```python
from build123d import *

# Parameters (mm, degrees)
SKETCH1_R           = 0.7874
BOSS_EXTRUDE1_DEPTH = 0.89
FILLET1_R           = 0.1


with BuildPart() as part:
    # Sketch1 → Boss-Extrude1 (new body)
    with BuildSketch(Plane(origin=(0, 0, 0), x_dir=(0, 0, -1), z_dir=(1, 0, 0))):
        with BuildLine():
            Line((-9.372828774, -0.73517355), (-7.483771729, 0.565616411))
            ThreePointArc((-7.483771729, 0.565616411), (-6.708837054, 2.194029076), (-7.731616452, 3.679348524))
            Line((-7.731616452, 3.679348524), (-9.134018919, 4.346728677))
            ThreePointArc((-9.134018919, 4.346728677), (6.441225552, -7.799677249), (-2.541446831, 9.791087775))
            Line((-2.541446831, 9.791087775), (-2.151242771, 8.287801467))
            ThreePointArc((-2.151242771, 8.287801467), (-0.886078684, 7.002651136), (0.859476194, 7.45574021))
            Line((0.859476194, 7.45574021), (2.493954423, 9.06479955))
            ThreePointArc((2.493954423, 9.06479955), (2.616717918, 9.131670791), (2.756271382, 9.123456835))
            ThreePointArc((2.756271382, 9.123456835), (5.588056342, -6.766575002), (-9.480022186, -0.981669875))
            ThreePointArc((-9.480022186, -0.981669875), (-9.461703842, -0.843080275), (-9.372828774, -0.73517355))
        make_face()
        with Locations((-8.506551123, 2.050935853)):
            Circle(SKETCH1_R, mode=Mode.SUBTRACT)
        with Locations((-0.405687887, 8.740890535)):
            Circle(SKETCH1_R, mode=Mode.SUBTRACT)
    extrude(amount=BOSS_EXTRUDE1_DEPTH)

    # Fillet1
    fillet1_edges = [part.edges().sort_by_distance(p)[0] for p in [
        (0.89, 2.194029076, 6.708837054),
        (0.89, 4.0130386, 8.432817685),
        (0.89, -7.799677249, -6.441225552),
        (0.89, 9.039444621, 2.346344801),
        (0.89, 2.050935853, 9.293951123),
        (0.89, 7.002651136, 0.886078684),
        (0.89, 8.740890535, 1.193087887),
        (0.89, 8.26026988, -1.676715309),
        (0.89, 9.131670791, -2.616717918),
        (0.89, -6.766575002, -5.588056342),
        (0.89, -0.843080275, 9.461703842),
        (0.89, -0.08477857, 8.428300251),
    ]]
    fillet(fillet1_edges, radius=FILLET1_R)


solid = part.part
```
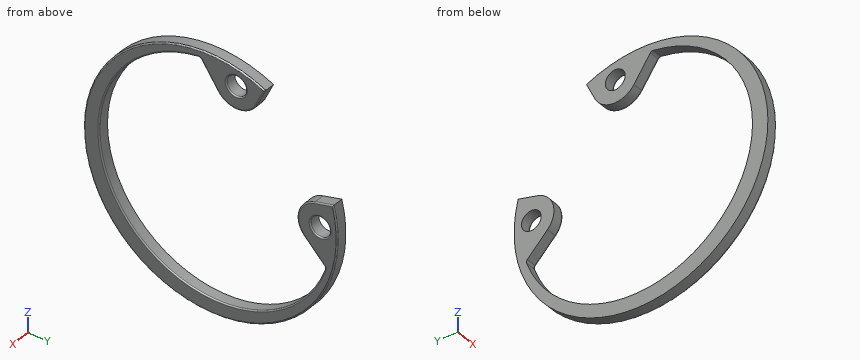
Design review of the part built by this model. Coordinates are the model's own, in mm. Coordinates: 2 decimals unless noted, no trailing zeros. Loops run counter-clockwise (first coordinate to the right, second up) from the corner with the lowest first, then second, coordinate; pieces in that order, holes last. Notation, with made-up numbers: (68.25, -4) - (117.25, -4) arc R36 ccw to (117.25, 35) - close; hole circle Ø9 at (42.5, -4). An arc over 180 degrees is marked (long way). Use CSV: the item, a comma, the result in double quotes. Start each with the question number.
1) For pin 1 Ø2 at (y, z) = (-7.5, 4.5) entering from +X, flat-tipped, find the tip position at first contact; note if it passes through.
2) Consider section B-B on z = 0. Give the number of separate pieces and of enclosed holes in the cut face, then the cut area to 3 significant figures.
3) Wall thickness on L1, parallel to Z at x = 0.4, y = 2.75; L2, parallel to Y at x = 0.65, z = -3.5; L3, parallel to Y at x = 0.1, z = -6.5: over which ranges is each line inside the solid? List them lowest first. Write a range as from..to.
4) Consider section A-A on x = 0.55. Write out the cut boundary in (y, z), then the cut area to 3 significant figures.
Geometry says:
1,pin 1,"x = 0.89"
2,separate pieces,"3"
2,enclosed holes,"0"
2,area,"2.67 mm^2"
3,L1,"-9.73..-8.65, 6.84..8.14, 8.87..9.73"
3,L2,"-9.49..-8.07, 8.83..9.49"
3,L3,"-7.75..-5.9, 6.66..7.75"
4,outline,"(-0.98, 9.48) arc R0.25 cw to (-0.74, 9.37) - (0.57, 7.48) arc R1.8 ccw to (3.68, 7.73) - (4.35, 9.13) arc R10.12 ccw (long way) to (9.79, 2.54) - (8.29, 2.15) arc R1.8 ccw to (7.46, -0.86) - (9.06, -2.49) arc R0.25 cw to (9.12, -2.76) arc R9.27 cw (long way) to start; hole circle Ø1.57 at (2.05, 8.51); hole circle Ø1.57 at (8.74, 0.41)"
4,area,"63.1 mm^2"
